CAD build for the part. Positions are in the model's coordinates, mm. Face numbers are marked on the shaded views. A direction names the side the tool comes from. Give positions to 0.01 mm unless a question says otherwise; leave off trailing zeros. Order: outer loops, then holes, each group sorted by start corner. A loop starts at its lowest first (then second) coordinate and runs counter-clockwise, first axis right, second up. Notation, with made-up numbers: (44.25, 77.5) -> (51.25, 77.5) arc R29 cw to (51.25, 113.5) -> close; hole circle Ø8 at (68, 47). An arc over 180 degrees is marked (long way). Answer as CSV lines item,"result".
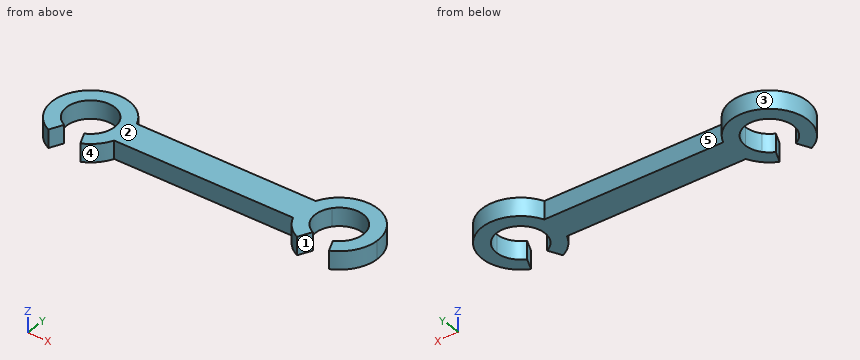
```python
from build123d import *

# Parameters (mm, degrees)
BOSS_EXTRU_1_DEPTH = 1.5


with BuildPart() as part:
    # Esquisse1 → Boss.-Extru.1 (new body)
    with BuildSketch(Plane.XY):
        with BuildLine():
            Line((-11.852378438, -2.900184919), (-11.345236523, -1.812615574))
            ThreePointArc((-11.345236523, -1.812615574), (-12.072600453, 1.235689207), (-8.9387505, 1.25))
            Line((-8.9387505, 1.25), (-7.554240336, 1.25))
            ThreePointArc((-7.554240336, 1.25), (-12.722774088, 2.302015498), (-11.852378438, -2.900184919))
        make_face()
        with BuildLine():
            ThreePointArc((-8.5, 0), (-8.612872686, -0.662382443), (-8.9387505, -1.25))
            Line((-8.9387505, -1.25), (-7.554240336, -1.25))
            ThreePointArc((-7.554240336, -1.25), (-7.364204174, -0.637796627), (-7.3, 0))
            ThreePointArc((-7.3, 0), (-7.364204174, 0.637796627), (-7.554240336, 1.25))
            Line((-7.554240336, 1.25), (-8.9387505, 1.25))
            ThreePointArc((-8.9387505, 1.25), (-8.612872686, 0.662382443), (-8.5, 0))
        make_face()
        with BuildLine():
            ThreePointArc((-7.3, 0), (-7.364204174, -0.637796627), (-7.554240336, -1.25))
            Line((-7.554240336, -1.25), (7.554240336, -1.25))
            ThreePointArc((7.554240336, -1.25), (7.3, 0), (7.554240336, 1.25))
            Line((7.554240336, 1.25), (-7.554240336, 1.25))
            ThreePointArc((-7.554240336, 1.25), (-7.364204174, 0.637796627), (-7.3, 0))
        make_face()
        with BuildLine():
            ThreePointArc((7.554240336, 1.25), (7.3, 0), (7.554240336, -1.25))
            Line((7.554240336, -1.25), (8.9387505, -1.25))
            ThreePointArc((8.9387505, -1.25), (8.5, 0), (8.9387505, 1.25))
            Line((8.9387505, 1.25), (7.554240336, 1.25))
        make_face()
        with BuildLine():
            ThreePointArc((13.7, 0), (11.137796627, 3.135795826), (7.554240336, 1.25))
            Line((7.554240336, 1.25), (8.9387505, 1.25))
            ThreePointArc((8.9387505, 1.25), (11.162382443, 1.887127314), (12.5, 0))
            ThreePointArc((12.5, 0), (12.186782892, -1.074599217), (11.345236523, -1.812615574))
            Line((11.345236523, -1.812615574), (11.852378438, -2.900184919))
            ThreePointArc((11.852378438, -2.900184919), (13.198852627, -1.719358747), (13.7, 0))
        make_face()
        with BuildLine():
            ThreePointArc((-8.9387505, -1.25), (-9.264310793, -1.572600453), (-9.654763477, -1.812615574))
            Line((-9.654763477, -1.812615574), (-9.147621562, -2.900184919))
            ThreePointArc((-9.147621562, -2.900184919), (-8.197984502, -2.222774088), (-7.554240336, -1.25))
            Line((-7.554240336, -1.25), (-8.9387505, -1.25))
        make_face()
        with BuildLine():
            Line((8.9387505, -1.25), (7.554240336, -1.25))
            ThreePointArc((7.554240336, -1.25), (8.197984502, -2.222774088), (9.147621562, -2.900184919))
            Line((9.147621562, -2.900184919), (9.654763477, -1.812615574))
            ThreePointArc((9.654763477, -1.812615574), (9.264310793, -1.572600453), (8.9387505, -1.25))
        make_face()
    extrude(amount=BOSS_EXTRU_1_DEPTH)


solid = part.part
```
1) Wall check: line 1 along X through (y, z) = (2.5, 1.3); line 2 along X through (y, z) = (-2.25, 1.4); line 3 along X through (y, z) = (1.5, 0.45). Give the ranges that are in metal, low to high. Write a range as [from, to].
Data:
line 1,"x = [-12.5, -8.5], [8.5, 12.5]"
line 2,"x = [-12.78, -11.55], [-9.45, -8.22], [8.22, 9.45], [11.55, 12.78]"
line 3,"x = [-13.33, -11.82], [-9.18, -7.67], [7.67, 9.18], [11.82, 13.33]"
2) Band-saw the part on A-A, the plane z = 0.4. Write the cut outline in (x, y), then the cut area to 3 significant figures.
Data:
outline,"(-11.85, -2.9) -> (-11.35, -1.81) arc R2 cw (long way) to (-9.65, -1.81) -> (-9.15, -2.9) arc R3.2 ccw to (-7.55, -1.25) -> (7.55, -1.25) arc R3.2 ccw to (9.15, -2.9) -> (9.65, -1.81) arc R2 cw (long way) to (11.35, -1.81) -> (11.85, -2.9) arc R3.2 ccw (long way) to (7.55, 1.25) -> (-7.55, 1.25) arc R3.2 ccw (long way) to start"
area,"70.7 mm2"
3) Band-saw the part on D-D, the plane x = -10.5. Write the cut outline in (y, z).
Data:
outline,"(2, 0) -> (3.2, 0) -> (3.2, 1.5) -> (2, 1.5) -> close"
4) Pull direction X, two halves, no side cores. Call the marked faces 1 and 2: pulls with the +X half, pulls with the -X half, needs draft (parallel to the pull), parting line crosses it, or undercut.
Data:
face 1,"undercut"
face 2,"needs draft"
5) Which spindle directions (+Z, -Z, +X, -X, +Y, -Y) get a long thin tool onto all of the face, cutting with end or side? Do the marked faces 3, 4 and 5. Say none if no direction does.
Data:
face 3,"+Z, -Z"
face 4,"+Z, -Z, -Y"
face 5,"+Z, -Z, +Y"
6) Band-saw the part on B-B, the plane y = 2.25. Write the cut outline in (x, z), then the cut area to 3 significant figures.
Data:
outline,"(-12.78, 0) -> (-8.22, 0) -> (-8.22, 1.5) -> (-12.78, 1.5) -> close; (8.22, 0) -> (12.78, 0) -> (12.78, 1.5) -> (8.22, 1.5) -> close"
area,"13.7 mm2"
7) Pin check, flat tips, straight feed: P1, Ø3, axis at x = -10.5, y = 0, coming from the +Z side; P2, Ø0.8, axis at x = -2.5, z = 1, coming from the +Y side. Stop position of each tip, or through.
Data:
P1,"passes through"
P2,"stops at y = 1.25"
8) Band-saw the part on C-C, the plane y = 1. Write the cut outline in (x, z).
Data:
outline,"(-13.54, 0) -> (-12.23, 0) -> (-12.23, 1.5) -> (-13.54, 1.5) -> close; (-8.77, 0) -> (8.77, 0) -> (8.77, 1.5) -> (-8.77, 1.5) -> close; (12.23, 0) -> (13.54, 0) -> (13.54, 1.5) -> (12.23, 1.5) -> close"
